from build123d import *

# Parameters (mm, degrees)
SKETCH1_W               = 80
SKETCH1_H               = 90
BOSS_EXTRUDE1_DEPTH     = 3
BOSS_EXTRUDE2_DEPTH     = 8
CUT_EXTRUDE1_DEPTH      = 114.670576668
SKETCH6_R               = 2
CUT_EXTRUDE3_DEPTH      = 25
MIRROR5_COPY_1_DEPTH    = 8
MIRROR5_COPY_2_DEPTH    = 114.670576668
MIRROR5_COPY_3_SKETCH_R = 2
MIRROR5_COPY_3_DEPTH    = 25
BOSS_EXTRUDE3_DEPTH     = 8
CUT_EXTRUDE2_DEPTH      = 25
SKETCH7_R               = 2
CUT_EXTRUDE4_DEPTH      = 25
SKETCH9_W               = 80
SKETCH9_H               = 90
BOSS_EXTRUDE7_DEPTH     = 35
CUT_EXTRUDE5_DEPTH      = 35
SKETCH11_W              = 13
SKETCH11_H              = 3
SKETCH11_W_2            = 10
SKETCH11_W_3            = 7
BOSS_EXTRUDE8_DEPTH     = 5
SKETCH12_W              = 9
SKETCH12_H              = 11
CUT_EXTRUDE6_DEPTH      = 46
SKETCH13_W              = 5
SKETCH13_H              = 12
CUT_EXTRUDE7_DEPTH      = 128.863208156
CUT_EXTRUDE8_DEPTH      = 1
CUT_EXTRUDE9_DEPTH      = 1
MIRROR7_COPY_1_DEPTH    = 1


with BuildPart() as part:
    # Sketch1 → Boss-Extrude1 (new body)
    with BuildSketch(Plane.XY):
        with Locations((40, 45)):
            Rectangle(SKETCH1_W, SKETCH1_H)
    extrude(amount=BOSS_EXTRUDE1_DEPTH)

    # Sketch2 → Boss-Extrude2 (add)
    with BuildSketch(Plane.XY.offset(3)):
        Polygon((0, 80), (10, 80), (10, 77), (2, 77), (2, 63), (10, 63), (10, 60), (0, 60), align=None)
    boss_extrude2 = extrude(amount=BOSS_EXTRUDE2_DEPTH)

    # Sketch3 → Cut-Extrude1 (cut, through all)
    with BuildSketch(Plane(origin=(0, 80, 0), x_dir=(1, 0, 0), z_dir=(0, 1, 0))):
        Polygon((10, -3), (2, -11), (10, -11), align=None)
    cut_extrude1 = extrude(amount=-CUT_EXTRUDE1_DEPTH, mode=Mode.SUBTRACT)

    # Sketch6 → Cut-Extrude3 (cut)
    with BuildSketch(Plane(origin=(2, 0, 0), x_dir=(0, 0, -1), z_dir=(1, 0, 0))):
        with Locations(Location((-7, 70, 0), (0, 0, 90))):
            Circle(SKETCH6_R)
    cut_extrude3 = extrude(amount=-CUT_EXTRUDE3_DEPTH, mode=Mode.SUBTRACT)

    # Mirror4: Boss-Extrude2, Cut-Extrude1, Cut-Extrude3 across plane
    add(boss_extrude2.mirror(Plane(origin=(40, 0, 0), x_dir=(0, 0, 1), z_dir=(1, 0, 0))))
    add(cut_extrude1.mirror(Plane(origin=(40, 0, 0), x_dir=(0, 0, 1), z_dir=(1, 0, 0))), mode=Mode.SUBTRACT)
    add(cut_extrude3.mirror(Plane(origin=(40, 0, 0), x_dir=(0, 0, 1), z_dir=(1, 0, 0))), mode=Mode.SUBTRACT)

    # Mirror5: Boss-Extrude2, Cut-Extrude1, Cut-Extrude3 across plane
    add(boss_extrude2.mirror(Plane(origin=(0, 45, 0), x_dir=(0, 0, 1), z_dir=(0, -1, 0))))
    add(cut_extrude1.mirror(Plane(origin=(0, 45, 0), x_dir=(0, 0, 1), z_dir=(0, -1, 0))), mode=Mode.SUBTRACT)
    add(cut_extrude3.mirror(Plane(origin=(0, 45, 0), x_dir=(0, 0, 1), z_dir=(0, -1, 0))), mode=Mode.SUBTRACT)

    # Mirror5 copy 1 sketch → Mirror5 copy 1 (add)
    with BuildSketch(Plane(origin=(80, 90, 3), x_dir=(-1, 0, 0), z_dir=(0, 0, 1))):
        Polygon((0, 80), (10, 80), (10, 77), (2, 77), (2, 63), (10, 63), (10, 60), (0, 60), align=None)
    extrude(amount=MIRROR5_COPY_1_DEPTH)

    # Mirror5 copy 2 sketch → Mirror5 copy 2 (cut, through all)
    with BuildSketch(Plane(origin=(80, 10, 0), x_dir=(-1, 0, 0), z_dir=(0, -1, 0))):
        Polygon((10, -3), (2, -11), (10, -11), align=None)
    extrude(amount=-MIRROR5_COPY_2_DEPTH, mode=Mode.SUBTRACT)

    # Mirror5 copy 3 sketch → Mirror5 copy 3 (cut)
    with BuildSketch(Plane(origin=(78, 90, 0), x_dir=(0, 0, -1), z_dir=(-1, 0, 0))):
        with Locations(Location((-7, 70, 0), (0, 0, 90))):
            Circle(MIRROR5_COPY_3_SKETCH_R)
    extrude(amount=-MIRROR5_COPY_3_DEPTH, mode=Mode.SUBTRACT)

    # Sketch4 → Boss-Extrude3 (add)
    with BuildSketch(Plane.XY.offset(3)):
        Polygon((30, 90), (50, 90), (50, 80), (47, 80), (47, 88), (33, 88), (33, 80), (30, 80), align=None)
    extrude(amount=BOSS_EXTRUDE3_DEPTH)

    # Sketch5 → Cut-Extrude2 (cut)
    with BuildSketch(Plane.ZY.offset(-30)):
        Polygon((3, 80), (11, 88), (11, 80), align=None)
    extrude(amount=-CUT_EXTRUDE2_DEPTH, mode=Mode.SUBTRACT)

    # Sketch7 → Cut-Extrude4 (cut)
    with BuildSketch(Plane.XZ.offset(-88)):
        with Locations(Location((40, 7, 0), (0, 0, 270))):
            Circle(SKETCH7_R)
    extrude(amount=-CUT_EXTRUDE4_DEPTH, mode=Mode.SUBTRACT)

    # Sketch9 → Boss-Extrude7 (add)
    with BuildSketch(Plane(origin=(0, 0, 0), x_dir=(-1, 0, 0), z_dir=(0, 0, -1))):
        with Locations((-40, 45)):
            Rectangle(SKETCH9_W, SKETCH9_H)
    extrude(amount=BOSS_EXTRUDE7_DEPTH)

    # Sketch10 → Cut-Extrude5 (cut)
    with BuildSketch(Plane.XY.offset(3)):
        Polygon((30, 87), (3, 87), (3, 80), (10, 80), (10, 77), (2, 77), (2, 63), (10, 63), (10, 60), (3, 60), (3, 30), (10, 30), (10, 27), (2, 27), (2, 13), (10, 13), (10, 10), (3, 10), (3, 0), (77, 0), (77, 10), (70, 10), (70, 13), (78, 13), (78, 27), (70, 27), (70, 30), (77, 30), (77, 60), (70, 60), (70, 63), (78, 63), (78, 77), (70, 77), (70, 80), (77, 80), (77, 87), (50, 87), (50, 80), (47, 80), (47, 88), (33, 88), (33, 80), (30, 80), align=None)
    extrude(amount=-CUT_EXTRUDE5_DEPTH, mode=Mode.SUBTRACT)

    # Sketch11 → Boss-Extrude8 (add)
    with BuildSketch(Plane.XY.offset(-32)):
        with Locations((8.5, 28.5)):
            Rectangle(SKETCH11_W, SKETCH11_H)
        with Locations((9.5, 51.5)):
            Rectangle(SKETCH11_W, SKETCH11_H)
        with Locations((40, 28.5)):
            Rectangle(SKETCH11_W_2, SKETCH11_H)
        with Locations((42.5, 51.5)):
            Rectangle(SKETCH11_W_3, SKETCH11_H)
    extrude(amount=BOSS_EXTRUDE8_DEPTH)

    # Sketch12 → Cut-Extrude6 (cut)
    with BuildSketch(Plane.XY.offset(-32)):
        with Locations((60.5, 63.5)):
            Rectangle(SKETCH12_W, SKETCH12_H)
    extrude(amount=-CUT_EXTRUDE6_DEPTH, mode=Mode.SUBTRACT)

    # Sketch13 → Cut-Extrude7 (cut, through all)
    with BuildSketch(Plane.XY.offset(-32)):
        with Locations((47.414473157, 64)):
            Rectangle(SKETCH13_W, SKETCH13_H)
    extrude(amount=-CUT_EXTRUDE7_DEPTH, mode=Mode.SUBTRACT)

    # Sketch14 → Cut-Extrude8 (cut)
    with BuildSketch(Plane.XZ.offset(-88)):
        Polygon((43.207910709, 5.692594599), (42.736201645, 9.124429466), (39.528290936, 10.431834868), (36.792089291, 8.307405401), (37.263798355, 4.875570534), (40.471709064, 3.568165132), align=None)
    extrude(amount=-CUT_EXTRUDE8_DEPTH, mode=Mode.SUBTRACT)

    # Sketch15 → Cut-Extrude9 (cut)
    with BuildSketch(Plane.ZY.offset(-78)):
        Polygon((9.993076519, 68.256012342), (10.006875875, 71.720086472), (7.013799356, 73.46407413), (4.006923481, 71.743987658), (3.993124125, 68.279913528), (6.986200644, 66.53592587), align=None)
    cut_extrude9 = extrude(amount=-CUT_EXTRUDE9_DEPTH, mode=Mode.SUBTRACT)

    # Mirror6: Cut-Extrude9 across plane
    add(cut_extrude9.mirror(Plane(origin=(40, 0, 0), x_dir=(0, 0, 1), z_dir=(1, 0, 0))), mode=Mode.SUBTRACT)

    # Mirror7: Cut-Extrude9 across plane
    add(cut_extrude9.mirror(Plane(origin=(0, 45, 0), x_dir=(0, 0, 1), z_dir=(0, -1, 0))), mode=Mode.SUBTRACT)

    # Mirror7 copy 1 sketch → Mirror7 copy 1 (cut)
    with BuildSketch(Plane(origin=(2, 90, 0), x_dir=(0, 0, 1), z_dir=(1, 0, 0))):
        Polygon((9.993076519, 68.256012342), (10.006875875, 71.720086472), (7.013799356, 73.46407413), (4.006923481, 71.743987658), (3.993124125, 68.279913528), (6.986200644, 66.53592587), align=None)
    extrude(amount=-MIRROR7_COPY_1_DEPTH, mode=Mode.SUBTRACT)


solid = part.part
Geometry: final body of the model. Coordinates: model frame, mm. A direction names the side the tool comes from. Coordinates: 2 decimals unless noted, no trailing zeros. Loops run counter-clockwise (first coordinate to the right, second up) from the corner with the lowest first, then second, coordinate; pieces in that order, holes last. Notation, with made-up numbers: M 37,-29 L 60,-29 A22 cw 60,4 Z; hole C 12.5,55.25 d7. An arc over 180 degrees is marked long. One line per item, written item: value. Start each with the question number.
1) Cut plane C-C (y = 20). Return loops of the section in (x, z).
2) Material intervals for L1, parallel to X at y = 50.5, z = -29.5; L2, parallel to Y at x = 75, z = -24.5; L3, parallel to X at y = 30.5, z = -6, sorted ascending. Write a range as from..to.
3) Pin query (flat end, axial travel): P1, Ø8, axis at x = 28, z = -9, coming from the -Y side; P2, Ø0.9, axis at x = 44, y = 51.5, coming from the +Z side; P3, Ø6.5, axis at x = 8.5, z = -16, coming from the -Y side. Return the tip coordinate at first contact, or that it passes through.
4) Reachability of faces 4 (the flat face through (47, 58, -33)), 5 (the flat face through (79, 69, 5)), 6 (the flat face through (38.2, 88.5, 9.4)), 7 (the flat face through (33, 84, -10)), 8 (the flat face through (74, 60, -11)) from +Z, -Z, +X, -X, +Y, -Y: full face, straight path, thin tool, end or side. Return the list, or none.
5) Cut plane A-A (x = 12.5). Return loops of the section in (y, z), then the cut area to 3 significant figures.
6) Draft query along Y for faces 1 (the flat face through (50, 84, -11)), 2 (the flat face through (3, 84, -14)), 3 (the flat face through (49, 80, -14)). Return one class per face: released by +Y, released by -Y, zero draft, split by the parting line, or undercut.
7) Cut plane B-B (y = 48.5). Return loops of the section in (x, z), then the cut area to 3 significant figures.
8) Cut plane D-D (x = 51.5). Return loops of the section in (y, z).
Evaluation:
1. outline: M 0,-35 L 80,-35 L 80,5 L 79,5 L 79,4 L 78,4 L 78,-32 L 2,-32 L 2,4 L 1,4 L 1,5 L 0,5 Z; M 0,9 L 1,9 L 1,10 L 2,10 L 2,11 L 0,11 Z; M 78,10 L 79,10 L 79,9 L 80,9 L 80,11 L 78,11 Z
2. L1: 0..16, 39..46, 77..80
2. L2: 10..13, 27..30, 60..63, 77..80, 87..90
2. L3: 0..3, 77..80
3. P1: y = 80
3. P2: z = -27
3. P3: y = 10
4. face 4: +Z, -Z
4. face 5: none
4. face 6: -Y
4. face 7: +Z, -Y
4. face 8: +Z
5. outline: M 0,-35 L 90,-35 L 90,3 L 87,3 L 87,-32 L 53,-32 L 53,-27 L 50,-27 L 50,-32 L 30,-32 L 30,-27 L 27,-27 L 27,-32 L 0,-32 Z
5. area: 405 mm^2
6. face 1: zero draft
6. face 2: undercut
6. face 3: released by -Y
7. outline: M 0,-35 L 80,-35 L 80,3 L 77,3 L 77,-32 L 3,-32 L 3,3 L 0,3 Z
7. area: 450 mm^2
8. outline: M 0,-35 L 90,-35 L 90,3 L 87,3 L 87,-32 L 0,-32 Z
